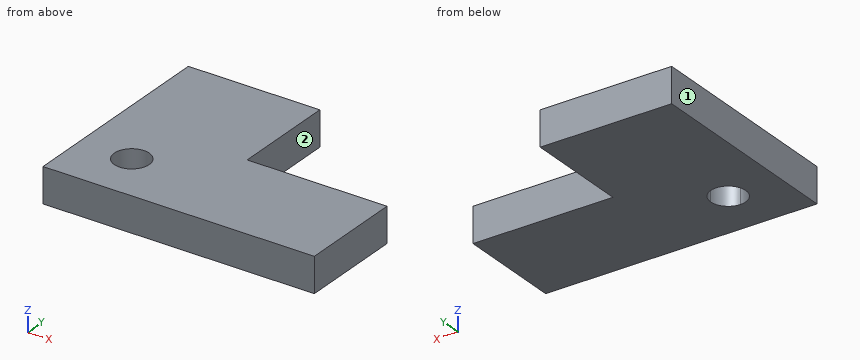
```python
from build123d import *

# Parameters (mm, degrees)
F1_DEPTH = 100
F3_DEPTH = 220.98


with BuildPart() as f1:
    # F0 (on Top) → F1 (new body)
    with BuildSketch(Plane.XY):
        Polygon((168.996112, -300), (168.996112, 0), (-207.003888, 0), (-207.003888, -600), (568.996112, -600), (568.996112, -300), align=None)
    extrude(amount=F1_DEPTH)

    # F2 (on face) → F3 (cut)
    with BuildSketch(Plane.XY.offset(100)):
        with BuildLine():
            ThreePointArc((-7.003888, -450), (-92.359227, -414.644661), (-57.003888, -500))
            ThreePointArc((-57.003888, -500), (-21.648549, -485.355339), (-7.003888, -450))
        make_face()
    extrude(amount=-F3_DEPTH, mode=Mode.SUBTRACT)


solid = f1.part
```
Geometry: final body of the model. Coordinates: model frame, mm. Face numbers are marked on the shaded views. A direction names the side the tool comes from. Coordinates: 2 decimals unless noted, no trailing zeros. Order: outer loops, then holes, each group sorted by start corner. A loop starts at its lowest first (then second) coordinate and runs counter-clockwise, first axis right, second up. Notation, with made-up numbers: M -21.75,-24.75 L 6.25,-24.75 A16 ccw 6.25,-14.75 Z; hole C -5,66 d11. An arc over 180 degrees is marked long. Answer as CSV lines item,"result".
Q1. Set-up query: the marked faces 1 and 2. Return all of +Z, -Z, +X, -X, +Y, -Y with unobstructed straight access to the full face (end or side cutting, diameter ignored); none if empty.
Answers:
face 1,"+Z, -Z, -X, +Y, -Y"
face 2,"+Z, -Z, +X, +Y"
Q2. First-contact query: P1, Ø12, axis at y = -283, z = 27, coming from the +X side; P2, Ø2, axis at x = 139, z = 34.5, coming from the +Y side. Flat tips, straight axial feed; report the tip coordinate or a pass-through.
Answers:
P1,"stops at x = 169"
P2,"stops at y = 0"
Q3. Section B-B on y = -472. Return the cut outline in (x, z), and give its area (3 significant figures).
Answers:
outline,"M -207,0 L -101.9,0 L -101.9,100 L -207,100 Z; M -12.1,0 L 569,0 L 569,100 L -12.1,100 Z"
area,"68,600 mm^2"
Q4. Section A-A on z = 87.5. Return the cut outline in (x, y).
Answers:
outline,"M -207,-600 L 569,-600 L 569,-300 L 169,-300 L 169,0 L -207,0 Z; hole C -57,-450 d100"
Q5. Section D-D on y = -97.5. Return the cut outline in (x, z).
Answers:
outline,"M -207,0 L 169,0 L 169,100 L -207,100 Z"
Q6. Section C-C on x = 479. Return the cut outline in (y, z), and give its area (3 significant figures).
Answers:
outline,"M -600,0 L -300,0 L -300,100 L -600,100 Z"
area,"30,000 mm^2"
Q7. Line query: probe 1 along X at (y, z) = (-450, 72); probe 2 along Y at (x, z) = (-59, 62.5); probe 3 along Y at (x, z) = (-49, 46). Output: solid intervals per line, ascending. Write a range as [from, to].
Answers:
probe 1,"x = [-207, -107], [-7, 569]"
probe 2,"y = [-600, -499.96], [-400.04, 0]"
probe 3,"y = [-600, -499.36], [-400.64, 0]"
